Design review of the part built by this model. Coordinates are the model's own, in mm. A direction names the side the tool comes from. Give positions to 0.01 mm unless a question says otherwise; leave off trailing zeros. Loops run counter-clockwise (first coordinate to the right, second up) from the corner with the lowest first, then second, coordinate; pieces in that order, holes last.
from build123d import *

# Parameters (mm, degrees)
BOSS_EXTRUDE1_DEPTH = 24
CHAMFER1_SIZE       = 0.4
FILLET1_R           = 0.3


with BuildPart() as part:
    # Sketch1 → Boss-Extrude1 (new, symmetric)
    with BuildSketch(Plane.XY):
        Polygon((0.9, -0.9), (0.9, -2.35), (-0.9, -2.35), (-0.9, -0.9), (-2.35, -0.9), (-2.35, 0.9), (-0.9, 0.9), (-0.9, 2.35), (0.9, 2.35), (0.9, 0.9), (2.35, 0.9), (2.35, -0.9), align=None)
    extrude(amount=BOSS_EXTRUDE1_DEPTH, both=True)

    # Chamfer1
    chamfer1_edges = [part.edges().sort_by_distance(p)[0] for p in [
        (0.9, -1.625, -24),
        (0, -2.35, -24),
        (1.625, 0.9, 24),
        (-0.9, -1.625, -24),
        (-1.625, -0.9, -24),
        (-2.35, 0, -24),
        (-1.625, 0.9, -24),
        (-0.9, 1.625, -24),
        (0, 2.35, -24),
        (0.9, 1.625, -24),
        (1.625, 0.9, -24),
        (2.35, 0, -24),
        (1.625, -0.9, -24),
        (0.9, 1.625, 24),
        (0, 2.35, 24),
        (-0.9, 1.625, 24),
        (-1.625, 0.9, 24),
        (-2.35, 0, 24),
        (-1.625, -0.9, 24),
        (-0.9, -1.625, 24),
        (0, -2.35, 24),
        (0.9, -1.625, 24),
        (1.625, -0.9, 24),
        (2.35, 0, 24),
    ]]
    chamfer(chamfer1_edges, length=CHAMFER1_SIZE)

    # Fillet1
    fillet1_edges = [part.edges().sort_by_distance(p)[0] for p in [
        (0.9, 0.9, 0),
        (-0.9, 0.9, 0),
        (-0.9, -0.9, 0),
        (0.9, -0.9, 0),
    ]]
    fillet(fillet1_edges, radius=FILLET1_R)


solid = part.part
Q1. Take a section at A-A (z = -18). Give the boundary of the cut face in (x, y), plus the area to 3 significant figures.
Results:
outline: (-2.35, -0.9) - (-1.2, -0.9) arc R0.3 cw to (-0.9, -1.2) - (-0.9, -2.35) - (0.9, -2.35) - (0.9, -1.2) arc R0.3 cw to (1.2, -0.9) - (2.35, -0.9) - (2.35, 0.9) - (1.2, 0.9) arc R0.3 cw to (0.9, 1.2) - (0.9, 2.35) - (-0.9, 2.35) - (-0.9, 1.2) arc R0.3 cw to (-1.2, 0.9) - (-2.35, 0.9) - close
area: 13.8 mm2
Q2. Tool access review of faces 1 (the face through (-0.9, -2, 0)), 2 (the face through (0.9, -2, 0)), 3 (the face through (0.9, 2, 0)), 4 (the face through (-2, 0.9, 0)), 5 (the face through (-2.35, 0, 0)): name each direction out of +Z, -Z, +X, -X, +Y, -Y from which nothing blocks a thin tool from reaching the whole face with its end or side.
Results:
face 1: +Z, -Z, -X, -Y
face 2: +Z, -Z, +X, -Y
face 3: +Z, -Z, +X, +Y
face 4: +Z, -Z, -X, +Y
face 5: +Z, -Z, -X, +Y, -Y
Q3. Insertion check: pin 1 (0.9 mm diameter, centred on y = -2, z = -8, fed in from -X); pin 2 (0.6 mm diameter, centred on x = 2, z = -3, fed in from -Y); pin 3 (0.6 mm diameter, centred on x = -1.5, z = -1, fed in from +Y). Each pin has a flat end and moves straight along its axis. Give the tip position at first contact, or say it passes through.
Results:
pin 1: stops at x = -0.9
pin 2: stops at y = -0.9
pin 3: stops at y = 0.9
Q4. Wall thickness on line 1 (X direction, y = 1.8, z = -18); line 2 (Z direction, x = -0.75, y = 1.2): over which ranges is each line inside the solid? List them lowest first.
Results:
line 1: x = -0.9 to 0.9
line 2: z = -23.75 to 23.75
